Answer from the drawing. Dimensions are ordinates in mm from the lowest x, y and z of the part. A direction names the side the tool comes from. Coordinates: 2 decimals unless noted, no trailing zeros. Order: outer loops, then holes, each group sorted by start corner. A loop starts at its lowest first (then second) coordinate and runs counter-clockwise, first axis right, second up. Notation, with made-up numbers: (64, -23) -> (108, -23) arc R36 cw to (108, 12) -> close; hole circle Ø10 at (24, 15). An arc over 180 degrees is marked (long way). Answer in a Markdown table with one row per item.
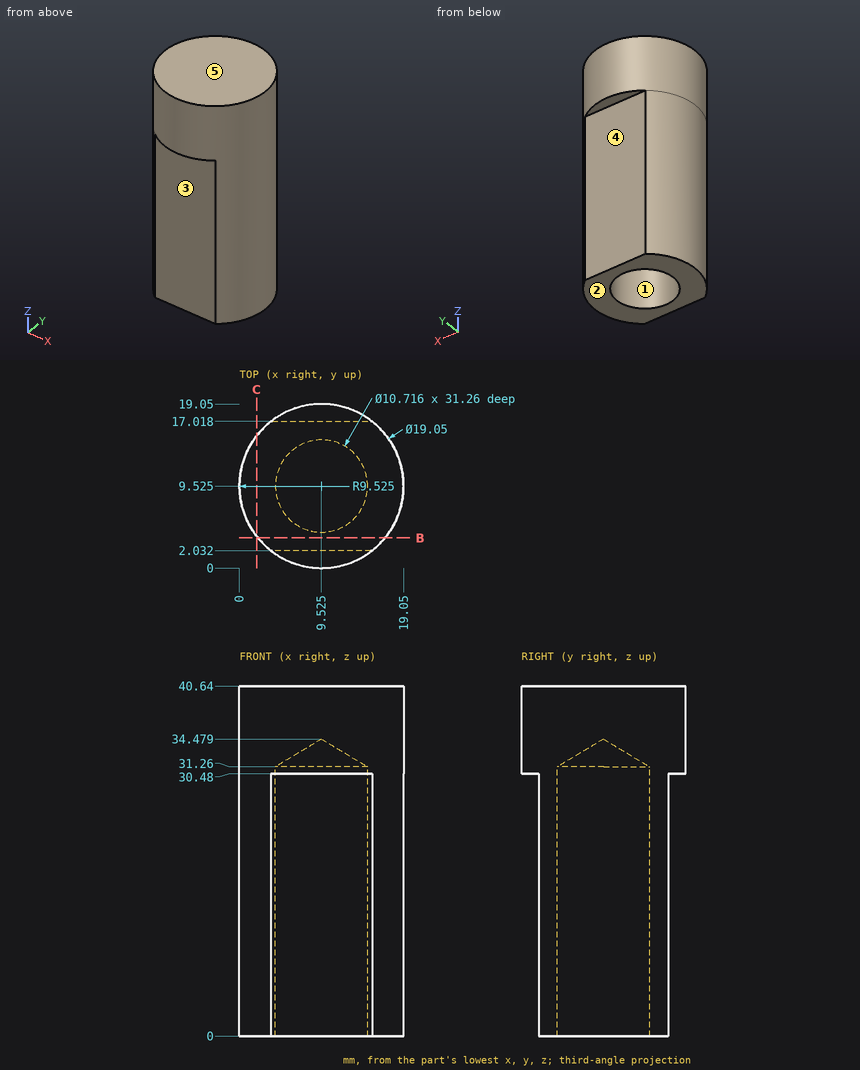
(1) Find the intervals of material crossed by line 1 along Y through (x, z) = (9.5, 25); line 2 along Y through (x, z) = (7.5, 19) (1 decimal); line 3 along X through (y, z) = (9, 3.5) (1 decimal), in increasing order. Write a range as from..to.
Check values:
| item | result |
|---|---|
| line 1 | 2.03..4.17, 14.88..17.02 |
| line 2 | 2..4.6, 14.5..17 |
| line 3 | 0..4.2, 14.9..19 |
(2) Flat-ended cylindrical pins translate along their axes: pin 1 (2 mm diameter, centred on x = 9.5, z = 17.5, fed in from -Y); pin 2 (1.6 mm diameter, centred on x = 9.5, y = 0.5, fed in from -Z); pin 3 (6 mm diameter, centred on x = 12, z = 22.5, fed in from +Y). Find the tip coordinate at first contact, or state that the pin passes through.
Check values:
| item | result |
|---|---|
| pin 1 | y = 2.03 |
| pin 2 | z = 30.48 |
| pin 3 | y = 17.02 |
(3) For a pull along X with two mould halves and no side action, classify the marked faces 1 and 2 as released by +X, released by -X, zero draft, split by the parting line, or undercut.
Check values:
| item | result |
|---|---|
| face 1 | undercut |
| face 2 | zero draft |
(4) Which of the six approach directions +Z, -Z, +X, -X, +Y, -Y give full straight-line access (tool end or side, diameter ignored) to the marked faces 3, 4 and 5?
Check values:
| item | result |
|---|---|
| face 3 | -Z, +X, -X, -Y |
| face 4 | -Z, +X, -X, +Y |
| face 5 | +Z, +X, -X, +Y, -Y |
(5) A cutting plane is placed at B-B, the plane y = 3.5. Determine the outline of the cut face in (x, z).
Check values:
| item | result |
|---|---|
| outline | (2.15, 0) -> (16.9, 0) -> (16.9, 40.64) -> (2.15, 40.64) -> close |
(6) A cutting plane is placed at C-C, the plane x = 2. Determine the outline of the cut face in (y, z) (1 decimal).
Check values:
| item | result |
|---|---|
| outline | (3.7, 0) -> (15.4, 0) -> (15.4, 40.6) -> (3.7, 40.6) -> close |
